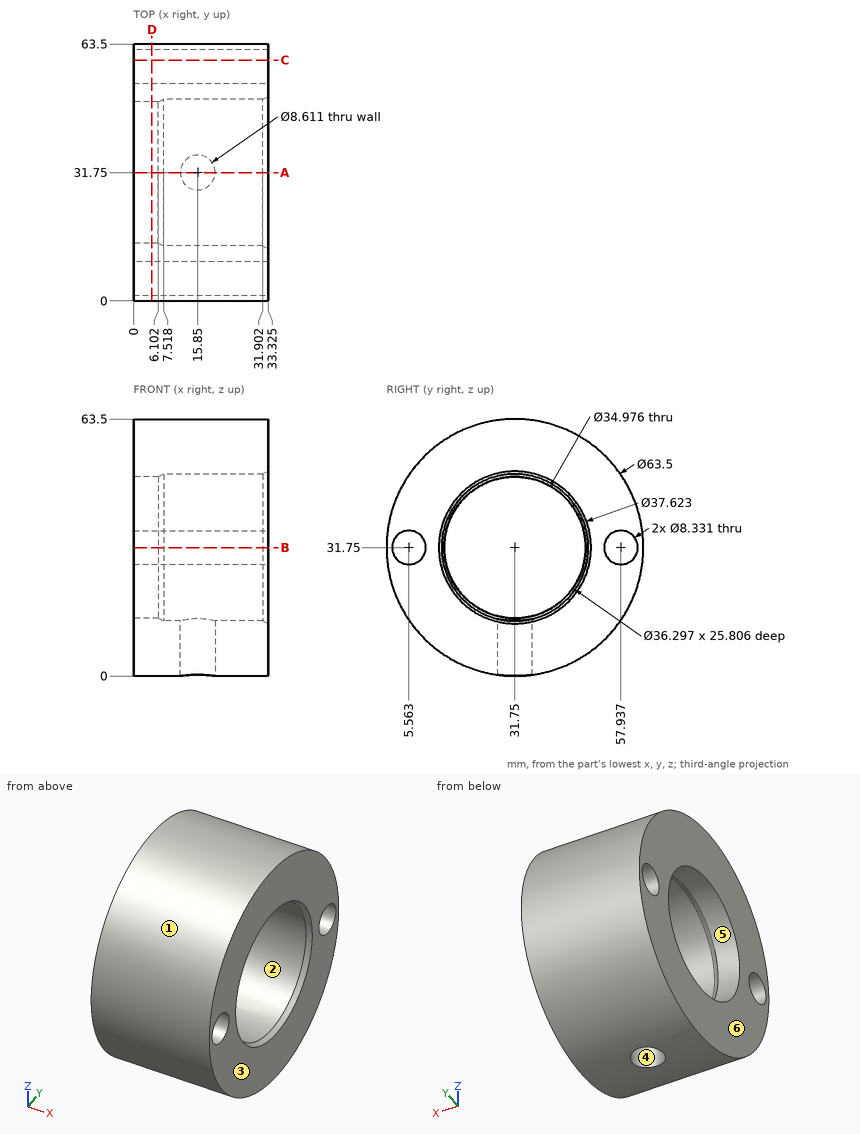
Part print with two shaded views. Sizes in mm from the minimum x, y, z corner. A direction names the side the tool comes from. Give positions to 0.01 mm unless a question says otherwise; leave off trailing zeros. Order: outer loops, then holes, each group sorted by start corner. A loop starts at its lowest first (then second) coordinate and runs counter-clockwise, first axis right, second up.
(1) Tool access for the marked faces 1 and 2: list every direction of +Z, -Z, +X, -X, +Y, -Y with a clear straight run to the whole face (end or side of a thin tool).
(2) Saw through at A-A, the plane y = 31.75. Give the cut face in (x, z) (1 decimal).
(3) Mould opens along X. For the marked faces 3, 4, 5 and 6 say: released by +X, released by -X, zero draft, split by the parting line, or undercut.
(4) Saw through at C-C, the plane y = 59.5. Give the cut face in (x, z) (1 decimal), then the cut area to 3 significant figures.
(5) Flat gauge pins, fed straight in: pin 1 (21 mm diameter, centred on y = 31.75, z = 31.75, fed in from +X); pin 2 (3 mm diameter, centred on x = 14, z = 6.5, fed in from -Y); pin 3 (12 mm diameter, centred on x = 8, z = 12.5, fed in from -Y); pin 4 (14 mm diameter, centred on x = 15.85, y = 31.75, fed in from +Z). Where does each tip first touch, or does it go through?
(6) Saw through at B-B, the plane z = 31.75. Give the cut face in (x, y) (1 decimal).
(7) Drill centre lines: L1, parallel to Y at x = 20, z = 31 (1 decimal); L2, parallel to Z at x = 25, y = 31; L3, parallel to Z at x = 2, y = 31. Where is each one in solid material? Low to high.
(8) Saw through at D-D, the plane x = 4.5. State how many separate pieces and enclosed holes the cut face has, then the cut area to 3 significant figures.
Results found:
1. face 1: +X, -X
1. face 2: +X
2. outline: (0, 0) - (11.5, 0) - (11.5, 13.6) - (7.5, 13.6) - (6.1, 14.3) - (0, 14.3) - close; (0, 49.2) - (6.1, 49.2) - (7.5, 49.9) - (31.9, 49.9) - (33.3, 50.6) - (33.3, 63.5) - (0, 63.5) - close; (20.2, 0) - (33.3, 0) - (33.3, 12.9) - (31.9, 13.6) - (20.2, 13.6) - close
3. face 3: released by +X
3. face 4: undercut
3. face 5: zero draft
3. face 6: released by -X
4. outline: (0, 16.3) - (33.3, 16.3) - (33.3, 27.9) - (0, 27.9) - close; (0, 35.6) - (33.3, 35.6) - (33.3, 47.2) - (0, 47.2) - close
4. area: 771 mm2
5. pin 1: passes through
5. pin 2: stops at y = 10.68
5. pin 3: stops at y = 2.9
5. pin 4: stops at z = 63.5
6. outline: (0, 0) - (33.3, 0) - (33.3, 1.4) - (0, 1.4) - close; (0, 9.7) - (33.3, 9.7) - (33.3, 12.9) - (31.9, 13.6) - (7.5, 13.6) - (6.1, 14.3) - (0, 14.3) - close; (0, 49.2) - (6.1, 49.2) - (7.5, 49.9) - (31.9, 49.9) - (33.3, 50.6) - (33.3, 53.8) - (0, 53.8) - close; (0, 62.1) - (33.3, 62.1) - (33.3, 63.5) - (0, 63.5) - close
7. L1: y = 0 to 1.5, 9.7 to 13.6, 49.9 to 53.8, 62 to 63.5
7. L2: z = 0.01 to 13.62, 49.88 to 63.49
7. L3: z = 0.01 to 14.28, 49.22 to 63.49
8. separate pieces: 1
8. enclosed holes: 3
8. area: 2,100 mm2
